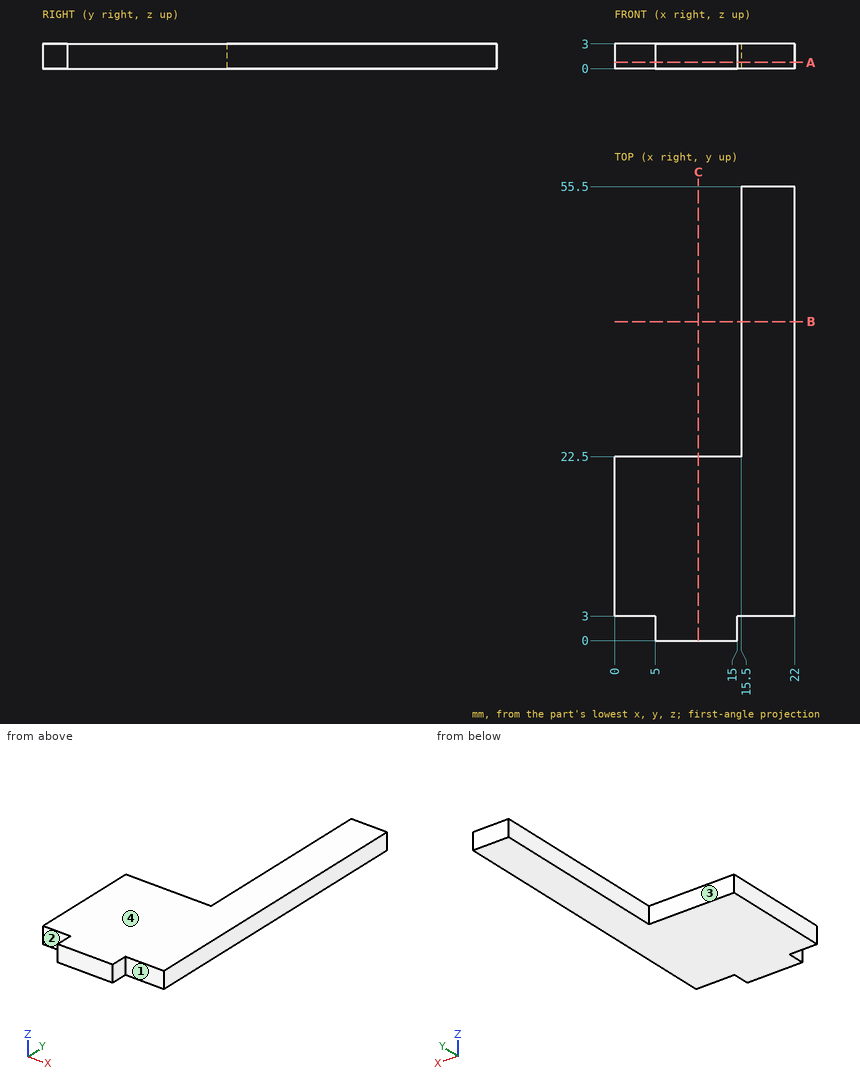
Answer from the drawing. Dimensions are ordinates in mm from the lowest x, y and z of the part. A direction names the side the tool comes from. Coordinates: 2 decimals unless noted, no trailing zeros. Order: outer loops, then holes, each group sorted by start corner. A loop starts at its lowest first (then second) coordinate and runs counter-clockwise, first axis right, second up. Notation, with made-up numbers: M 74,0 L 79,0 A12 ccw 79,10 Z; hole C 39,-33.75 d1. An arc over 180 degrees is marked long. Put each result on its own line as item: value. Start each with the question number.
Item 1: Given pin 1 Ø1.5 at (y, z) = (1.5, 1.5) entering from -X; pin 2 Ø1.5 at (x, z) = (20, 1) entering from -Y; pin 3 Ø1 at (y, z) = (45.5, 0.5) entering from -X, each flat-ended and moving along its own axis, determine where each tip first touches the part or whether it passes through.
Item 2: Consider probe 1 along Y at (x, z) = (13.5, 1.6); probe 2 along Y at (x, z) = (16.25, 1.95); probe 3 along X at (y, z) = (32.5, 2.8). Determine where each line is inside the solid, lowest interval first. Write a range as [from, to].
Item 3: Section C-C, the plane x = 10.25 is taken. Determine the outline of the cut face in (y, z).
Item 4: For the marked faces 1, 2, 3 and 4, determine the directions among +Z, -Z, +X, -X, +Y, -Y from which every point of the face is accessible in a straight line to the end or side of a thin tool.
Item 5: Section B-B, the plane y = 39 is taken. Determine the outline of the cut face in (x, z), plus the area to 3 significant figures.
Item 6: Section A-A, the plane z = 0.75 is taken. Determine the outline of the cut face in (x, y), plus the area to 4 significant figures.
Computed:
1. pin 1: stops at x = 5
1. pin 2: stops at y = 3
1. pin 3: stops at x = 15.5
2. probe 1: y = [0, 22.5]
2. probe 2: y = [3, 55.5]
2. probe 3: x = [15.5, 22]
3. outline: M 0,0 L 22.5,0 L 22.5,3 L 0,3 Z
4. face 1: +Z, -Z, +X, -Y
4. face 2: +Z, -Z, -X, -Y
4. face 3: +Z, -Z, -X, +Y
4. face 4: +Z, +X, -X, +Y, -Y
5. outline: M 15.5,0 L 22,0 L 22,3 L 15.5,3 Z
5. area: 19.5 mm2
6. outline: M 0,3 L 5,3 L 5,0 L 15,0 L 15,3 L 22,3 L 22,55.5 L 15.5,55.5 L 15.5,22.5 L 0,22.5 Z
6. area: 673.5 mm2
